from build123d import *

# Parameters (mm, degrees)
SKETCH1_W           = 193
SKETCH1_H           = 59
BOSS_EXTRUDE1_DEPTH = 6
SKETCH3_W           = 6
SKETCH3_H           = 15
SKETCH3_H_2         = 9
SKETCH3_H_3         = 12
CUT_EXTRUDE1_DEPTH  = 7
SKETCH4_W           = 199.10755054
SKETCH4_H           = 40.828336107
CUT_EXTRUDE2_DEPTH  = 7


with BuildPart() as part:
    # Sketch1 → Boss-Extrude1 (new body)
    with BuildSketch(Plane(origin=(0, 0, 0), x_dir=(1, 0, 0), z_dir=(0, 1, 0))):
        Rectangle(SKETCH1_W, SKETCH1_H)
    extrude(amount=BOSS_EXTRUDE1_DEPTH)

    # Sketch3 → Cut-Extrude1 (cut, through all)
    with BuildSketch(Plane(origin=(0, 0, 0), x_dir=(-1, 0, 0), z_dir=(0, -1, 0))):
        with Locations((79, 22)):
            Rectangle(SKETCH3_W, SKETCH3_H)
        with Locations((79, -22)):
            Rectangle(SKETCH3_W, SKETCH3_H)
        with Locations((79, 0)):
            Rectangle(SKETCH3_W, SKETCH3_H_2)
        with Locations((73, 0)):
            Rectangle(SKETCH3_W, SKETCH3_H_3)
    extrude(amount=-CUT_EXTRUDE1_DEPTH, mode=Mode.SUBTRACT)

    # Sketch4 → Cut-Extrude2 (cut, through all)
    with BuildSketch(Plane.XZ):
        with Locations((-141.775997492, -49.914168053)):
            Rectangle(SKETCH4_W, SKETCH4_H)
        with Locations((-107.998219714, -49.914168053)):
            Rectangle(SKETCH4_W, SKETCH4_H)
    cut_extrude2 = extrude(amount=-CUT_EXTRUDE2_DEPTH, mode=Mode.SUBTRACT)

    # Mirror1: Cut-Extrude2 across plane
    add(cut_extrude2.mirror(Plane.XY), mode=Mode.SUBTRACT)

    # Mirror2: Cut-Extrude2 across plane
    add(cut_extrude2.mirror(Plane(origin=(0, 0, 0), x_dir=(0, 0, 1), z_dir=(1, 0, 0))), mode=Mode.SUBTRACT)


solid = part.part
Geometry: final body of the model. Coordinates: model frame, mm. A direction names the side the tool comes from. Give positions to 0.01 mm unless a question says otherwise; leave off trailing zeros. Write each loop counter-clockwise with the first axis right and the second up, starting at its lowest first coordinate (ties: lowest second). Pieces come first, ordered by that corner, then holes. Notation, with made-up numbers: M 56,27.5 L 78,27.5 A16 cw 78,38.5 Z; hole C -22.75,48.5 d1. An arc over 180 degrees is marked long. Answer in a Markdown table with one row per item. Add a question column.
(1) Section B-B on y = 1.5. Return loops of the section in (x, z), and give its area (3 significant figures).
(2) Ray query, line 1 (X direction, y = 4.4, z = 16.5); line 2 (X direction, y = 0.95, z = -3.5); line 3 (Z direction, x = -73.5, y = 1.45). Return the intervals inside material, ascending.
(3) First-contact query: pin 1 (1.8 mm diameter, centred on x = -79.5, y = 3, fed in from +Z). Flat tip, straight axial feed; report the tip coordinate or a pass-through.
(4) Reachability of faces 1 (the flat face through (-82, 3, 0)), 2 (the flat face through (-79, 3, 14.5)), 3 (the flat face through (-1, 0, 0)), 4 (the flat face through (-1, 6, 0)), 5 (the flat face through (-82, 3, -22)) from +Z, -Z, +X, -X, +Y, -Y: full face, straight path, thin tool, end or side. Return the list, or none.
(5) Section A-A on z = 18. Return loops of the section in (x, y).
(6) Mould query, pull axis X, two halves, no side actions, for faces 6 (the flat face through (9, 3, 29.5)), 7 (the flat face through (-79, 3, 4.5)), 8 (the flat face through (-76, 3, -22)), 9 (the flat face through (-96.5, 3, 0)). Classes: +X half, -X half, draft (parallel to the pull), parting line (faces both ways), or undercut.
Result set:
| question | item | result |
|---|---|---|
| 1 | outline | M -96.5,-29.5 L -82,-29.5 L -82,-14.5 L -76,-14.5 L -76,-29.5 L 96.5,-29.5 L 96.5,29.5 L -76,29.5 L -76,14.5 L -82,14.5 L -82,29.5 L -96.5,29.5 Z; hole M -82,-4.5 L -76,-4.5 L -76,-6 L -70,-6 L -70,6 L -76,6 L -76,4.5 L -82,4.5 Z |
| 1 | area | 11,100 mm^2 |
| 2 | line 1 | x = -96.5 to -82, -76 to 96.5 |
| 2 | line 2 | x = -96.5 to -82, -70 to 96.5 |
| 2 | line 3 | z = -29.5 to -6, 6 to 29.5 |
| 3 | pin 1 | stops at z = 14.5 |
| 4 | face 1 | +Y, -Y |
| 4 | face 2 | +Z, +Y, -Y |
| 4 | face 3 | +Z, -Z, +X, -X, -Y |
| 4 | face 4 | +Z, -Z, +X, -X, +Y |
| 4 | face 5 | -Z, +Y, -Y |
| 5 | outline | M -96.5,0 L -82,0 L -82,6 L -96.5,6 Z; M -76,0 L 96.5,0 L 96.5,6 L -76,6 Z |
| 6 | face 6 | draft |
| 6 | face 7 | undercut |
| 6 | face 8 | undercut |
| 6 | face 9 | -X half |
